Work out the finished part from the listing and answer in its coordinate system (mm). A direction names the side the tool comes from. Give positions to 0.01 mm unless a question says otherwise; leave off trailing zeros. Write each loop counter-clockwise with the first axis right and the second up, starting at its lowest first coordinate (ties: lowest second). Pieces come first, ordered by that corner, then holes. Notation, with made-up numbers: (-12.75, 35.25) -> (13.25, 35.25) arc R32 cw to (13.25, 65.25) -> close; hole circle Ø7 at (89.5, 53). An arc over 180 degrees is marked (long way). Use a Markdown table: item, result. Add a question column.
Q1. For a pull along Z with two mould halves and no side action, classify faces 4 (the face through (1, -5, -5)), 5 (the face through (-1.207, -7.26, 0.604)), 6 (the face through (-2, -6.5, -1)), 7 (the face through (-0.79, -7.83, 1.79)) as pulls with the +Z half, pulls with the -Z half, needs draft (parallel to the pull), parting line crosses it, or undercut.
Q2. Section D-D, the plane z = 0 is taken. Give the vertices of the cut face in (x, y), plus the area to 3 significant figures.
Q3. Consider line 1 (X direction, y = -7.6, z = 0.5); line 2 (Y direction, x = 1.45, z = 0); line 3 (X direction, y = 2.5, z = -2.75). Determine where each line is inside the solid, lowest interval first.
Q4. Section C-C, the plane x = -3 is taken. Give the vertices of the cut face in (y, z), plus the area to 3 significant figures.
Q5. Each of these flat-tipped pins is pushed along its axis until it touches: pin 1 Ø5 at (y, z) = (-1.5, -2.5) entering from -X; pin 2 Ø1.2 at (x, y) = (0.5, -6.5) entering from +Z; pin 3 Ø1 at (x, z) = (1.5, 4) entering from -Y. Where does it stop, or does it pass through?
Q6. Section B-B, the plane y = -3.5 is taken. Give the vertices of the cut face in (x, z).
Q7. Section A-A, the plane x = 1.25 is taken. Give the vertices of the cut face in (y, z).
Q8. For faces 1 (the face through (0, -7, 2.5)), 2 (the face through (0, -3, -2)), 3 (the face through (-4, -7, -1)), determine the directions among +Z, -Z, +X, -X, +Y, -Y from which every point of the face is accessible in a straight line to the end or side of a thin tool.
from build123d import *

# Parameters (mm, degrees)
SKETCH_1_R          = 3
EXTRUDE_1_DEPTH     = 2.5
SKETCH_2_W          = 6.5
SKETCH_2_H          = 10
SKETCH_2_R          = 0.8
EXTRUDE_2_DEPTH     = 1.5
SKETCH_5_W          = 6.5
SKETCH_5_H          = 2.5
CUT_EXTRUDE_1_DEPTH = 2.5
CUT_EXTRUDE_2_REACH = 13.456
FILLET_1_R          = 0.2
FILLET_2_R          = 0.2
CHAMFER_1_SIZE      = 0.2


with BuildPart() as part:
    # 草图1 → 凸台-拉伸1 (new body)
    with BuildSketch(Plane(origin=(0, 0, 0), x_dir=(0, 0, -1), z_dir=(1, 0, 0))):
        with BuildLine():
            Line((-5, 0), (-5, -8))
            Line((-5, -8), (5, -8))
            Line((5, -8), (5, 0))
            ThreePointArc((5, 0), (0, 5), (-5, 0))
        make_face()
        Circle(SKETCH_1_R, mode=Mode.SUBTRACT)
    extrude(amount=EXTRUDE_1_DEPTH)

    # 草图2 → 凸台-拉伸2 (add)
    with BuildSketch(Plane.XZ.offset(8)):
        with Locations((-0.75, 0)):
            Rectangle(SKETCH_2_W, SKETCH_2_H)
        with Locations(Location((-2, 0.5, 0), (0, 0, 270))):
            Circle(SKETCH_2_R, mode=Mode.SUBTRACT)
        with Locations(Location((-2, -3, 0), (0, 0, 270))):
            Circle(SKETCH_2_R, mode=Mode.SUBTRACT)
    extrude(amount=-EXTRUDE_2_DEPTH)

    # 草图5 → 切除-拉伸1 (cut)
    with BuildSketch(Plane.XZ.offset(8)):
        with Locations((-0.75, 3.75)):
            Rectangle(SKETCH_5_W, SKETCH_5_H)
    extrude(amount=-CUT_EXTRUDE_1_DEPTH, mode=Mode.SUBTRACT)

    # 草图6 → 切除-拉伸2 (cut, up to next)
    with BuildSketch(Plane.ZY.offset(4), mode=Mode.PRIVATE) as cut_extrude_2_sk1:
        with BuildLine():
            Line((2.897366596, -6), (3.27705392, -6))
            Line((3.27705392, -6), (3.27705392, -8.325127743))
            Line((3.27705392, -8.325127743), (1, -8.325127743))
            Line((1, -8.325127743), (1, -8))
            ThreePointArc((1, -8), (2.378404875, -7.407669683), (2.897366596, -6))
        make_face()
    cut_extrude_2_tool1 = extrude(cut_extrude_2_sk1.sketch, amount=-CUT_EXTRUDE_2_REACH, mode=Mode.PRIVATE) & part.part
    add(cut_extrude_2_tool1.solids().sort_by_distance((-4, -7.575754, 2.569334))[0], mode=Mode.SUBTRACT)

    # 圆角1
    fillet_1_edges = [part.edges().sort_by_distance(p)[0] for p in [
        (0, -6.5, -1.25),
    ]]
    fillet(fillet_1_edges, radius=FILLET_1_R)

    # 圆角2
    fillet_2_edges = [part.edges().sort_by_distance(p)[0] for p in [
        (2.5, -4, -5),
        (-2.1, -6.5, -5),
        (-4, -7.25, -5),
        (2.5, 5, 0),
        (-4, -6.5, -1.25),
        (1.25, -5.5, 5),
        (-2.1, -6.5, 2.5),
        (1.25, -5.5, 2.5),
        (2.5, -6.383095189, 2.5),
        (2.5, -5.5, 3.75),
        (0, -5.5, 3.75),
        (0, -2.75, 5),
        (0, 5, 0),
        (-4, -8, -2),
        (2.5, -8, -2),
        (-0.75, -7.266190379, 2.5),
        (2.5, -7.806716397, 1.834936608),
        (-4, -7.806716397, 1.834936608),
        (2.5, -2.75, 5),
        (-0.75, -8, -5),
        (0, -5.9, 2.5),
        (0, -3.15, -5),
        (-0.058578644, -6.441421356, -5),
        (-0.058578644, -6.441421356, 2.5),
    ]]
    fillet(fillet_2_edges, radius=FILLET_2_R)

    # 倒角1
    chamfer_1_edges = [part.edges().sort_by_distance(p)[0] for p in [
        (0, 0, 3),
        (2.5, 0, 3),
    ]]
    chamfer(chamfer_1_edges, length=CHAMFER_1_SIZE)


solid = part.part
Result set:
| question | item | result |
|---|---|---|
| 1 | face 4 | pulls with the -Z half |
| 1 | face 5 | undercut |
| 1 | face 6 | needs draft |
| 1 | face 7 | pulls with the +Z half |
| 2 | outline | (-4, -7.8) arc R0.2 ccw to (-3.8, -8) -> (-2.62, -8) -> (-2.62, -6.5) -> (-3.8, -6.5) arc R0.2 ccw to (-4, -6.7) -> close; (-1.38, -8) -> (2.3, -8) arc R0.2 ccw to (2.5, -7.8) -> (2.5, -3.2) -> (2.3, -3) -> (0.2, -3) -> (0, -3.2) -> (0, -6.3) arc R0.2 cw to (-0.2, -6.5) -> (-1.38, -6.5) -> close; (0, 3.2) -> (0.2, 3) -> (2.3, 3) -> (2.5, 3.2) -> (2.5, 4.8) arc R0.2 ccw to (2.3, 5) -> (0.2, 5) arc R0.2 ccw to (0, 4.8) -> close |
| 2 | area | 21.5 mm2 |
| 3 | line 1 | x = -4 to -2.8, -1.2 to 2.5 |
| 3 | line 2 | y = -8 to -3, 3 to 5 |
| 3 | line 3 | x = 0 to 2.5 |
| 4 | outline | (-8, -4.8) arc R0.2 ccw to (-7.8, -5) -> (-6.7, -5) arc R0.2 ccw to (-6.5, -4.8) -> (-6.5, 2.3) arc R0.2 ccw to (-6.7, 2.5) -> (-7.2, 2.5) arc R0.2 ccw to (-7.32, 2.45) arc R1.9 ccw to (-8, 1) -> close |
| 4 | area | 10.9 mm2 |
| 5 | pin 1 | stops at x = 0 |
| 5 | pin 2 | stops at z = 2.5 |
| 5 | pin 3 | stops at y = -5.5 |
| 6 | outline | (0, -4.8) arc R0.2 ccw to (0.2, -5) -> (2.3, -5) arc R0.2 ccw to (2.5, -4.8) -> (2.5, 4.8) arc R0.2 ccw to (2.3, 5) -> (0.2, 5) arc R0.2 ccw to (0, 4.8) -> close |
| 7 | outline | (-8, -4.8) arc R0.2 ccw to (-7.8, -5) -> (0, -5) arc R5 ccw to (0, 5) -> (-5.3, 5) arc R0.2 ccw to (-5.5, 4.8) -> (-5.5, 2.7) arc R0.2 cw to (-5.7, 2.5) -> (-7.2, 2.5) arc R0.2 ccw to (-7.32, 2.45) arc R1.9 ccw to (-8, 1) -> close; hole circle Ø6 at (0, 0) |
| 8 | face 1 | +Z, +X, -X, -Y |
| 8 | face 2 | +Z, -Z, -X, +Y |
| 8 | face 3 | +Z, -Z, -X, +Y, -Y |
